```python
from build123d import *

# Parameters (mm, degrees)
SKETCH1_W                    = 38.1
SKETCH1_H                    = 53.34
BOSS_EXTRUDE1_DEPTH          = 1.5875
EDGE_FLANGE1_STRIP_W         = 9.525
EDGE_FLANGE1_STRIP_H         = 1.5875
EDGE_FLANGE1_STRIP_CUT_DEPTH = 38.1
EDGE_FLANGE1_DEPTH           = 38.1
CUT_EXTRUDE1_REACH           = 40.731
SKETCH9_R                    = 2.54
CUT_EXTRUDE2_REACH           = 61.758
SKETCH11_R                   = 2.54


# Sheet-metal steps are written as plain solids
with BuildPart() as part:
    # Sketch1 → Boss-Extrude1 (new body)
    with BuildSketch(Plane(origin=(0, 0, 0), x_dir=(1, 0, 0), z_dir=(0, 1, 0))):
        Rectangle(SKETCH1_W, SKETCH1_H)
    extrude(amount=BOSS_EXTRUDE1_DEPTH)

    # Edge-Flange1 strip (across the edge) → Edge-Flange1 strip cut (cut)
    with BuildSketch(Plane(origin=(19.05, 0, 26.67), x_dir=(0, 0, -1), z_dir=(-1, 0, 0))):
        with Locations((-1.5875, -0.79375)):
            Rectangle(EDGE_FLANGE1_STRIP_W, EDGE_FLANGE1_STRIP_H)
    extrude(amount=EDGE_FLANGE1_STRIP_CUT_DEPTH, mode=Mode.SUBTRACT)

    # Edge-Flange1 section (across the edge) → Edge-Flange1 (add)
    with BuildSketch(Plane(origin=(19.05, 0, 26.67), x_dir=(0, 0, -1), z_dir=(-1, 0, 0))):
        with BuildLine():
            Line((0, 1.5875), (0, 19.05))
            Line((0, 19.05), (1.5875, 19.05))
            Line((1.5875, 19.05), (1.5875, 1.5875))
            ThreePointArc((1.5875, 1.5875), (2.052467985, 0.464967985), (3.175, 0))
            Line((3.175, 0), (3.175, -1.5875))
            ThreePointArc((3.175, -1.5875), (0.92993597, -0.65756403), (0, 1.5875))
        make_face()
    extrude(amount=EDGE_FLANGE1_DEPTH)

    # Sketch9 → Cut-Extrude1 (cut, up to next)
    with BuildSketch(Plane(origin=(0, 1.5875, 0), x_dir=(1, 0, 0), z_dir=(0, 1, 0)), mode=Mode.PRIVATE) as cut_extrude1_sk1:
        with Locations(Location((9.813099354, 13.0175, 0), (0, 0, 270))):
            Circle(SKETCH9_R)
    cut_extrude1_tool1 = extrude(cut_extrude1_sk1.sketch, amount=-CUT_EXTRUDE1_REACH, mode=Mode.PRIVATE) & part.part
    # Sketch9 → Cut-Extrude1 (cut, up to next)
    with BuildSketch(Plane(origin=(0, 1.5875, 0), x_dir=(1, 0, 0), z_dir=(0, 1, 0)), mode=Mode.PRIVATE) as cut_extrude1_sk2:
        with Locations(Location((-9.236900646, 13.0175, 0), (0, 0, 270))):
            Circle(SKETCH9_R)
    cut_extrude1_tool2 = extrude(cut_extrude1_sk2.sketch, amount=-CUT_EXTRUDE1_REACH, mode=Mode.PRIVATE) & part.part
    add(cut_extrude1_tool1.solids().sort_by_distance((9.813099, 1.5875, -13.0175))[0], mode=Mode.SUBTRACT)
    add(cut_extrude1_tool2.solids().sort_by_distance((-9.236901, 1.5875, -13.0175))[0], mode=Mode.SUBTRACT)

    # Sketch11 → Cut-Extrude2 (cut, up to next)
    with BuildSketch(Plane.XY.offset(26.67), mode=Mode.PRIVATE) as cut_extrude2_sk1:
        with Locations((-9.398, -9.398)):
            Circle(SKETCH11_R)
    cut_extrude2_tool1 = extrude(cut_extrude2_sk1.sketch, amount=-CUT_EXTRUDE2_REACH, mode=Mode.PRIVATE) & part.part
    # Sketch11 → Cut-Extrude2 (cut, up to next)
    with BuildSketch(Plane.XY.offset(26.67), mode=Mode.PRIVATE) as cut_extrude2_sk2:
        with Locations((9.398, -9.398)):
            Circle(SKETCH11_R)
    cut_extrude2_tool2 = extrude(cut_extrude2_sk2.sketch, amount=-CUT_EXTRUDE2_REACH, mode=Mode.PRIVATE) & part.part
    add(cut_extrude2_tool1.solids().sort_by_distance((-9.398, -9.398, 26.67))[0], mode=Mode.SUBTRACT)
    add(cut_extrude2_tool2.solids().sort_by_distance((9.398, -9.398, 26.67))[0], mode=Mode.SUBTRACT)


solid = part.part
```
Input: part model. Units: mm. Frame: model coordinates. A direction names the side the tool comes from. Coordinates: 2 decimals unless noted, no trailing zeros. Loops run counter-clockwise (first coordinate to the right, second up) from the corner with the lowest first, then second, coordinate; pieces in that order, holes last. Notation, with made-up numbers: M 14.25,89 L 45.25,89 A18 cw 45.25,111 Z; hole C 62,16.25 d11. An arc over 180 degrees is marked long. Use a Markdown table: item, result. Add a question column.
1) Draft query along X for faces 3 (the cylindrical face through (-10.782, 0.805, -15.033)), 4 (the flat face through (0, -19.05, 26)), 5 (the flat face through (-19.05, 0.4, 7.8)), 6 (the cylindrical face through (11.821, -8.635, 25.887)). Return one class per face: +X half, -X half, draft (parallel to the pull), parting line (faces both ways), or undercut.
2) Set-up query: faces 1 (the flat face through (0, -10, 25.083)), 2 (the flat face through (0, 1, -26.67)). Return all of +Z, -Z, +X, -X, +Y, -Y with unobstructed straight access to the full face (end or side cutting, diameter ignored); none if empty.
3) Pin query (flat end, axial travel): P1, Ø1, axis at x = 15, z = 17.5, coming from the -Y side; P2, Ø5, axis at x = -6.5, y = -13, coming from the -Z side. Return the tip coordinate at first contact, or that it passes through.
4) Section B-B, the plane y = -10.75. Return the cut outline in (x, z).
5) Section D-D, the plane z = 0. Return the cut outline in (x, y).
6) Line query: L1, parallel to Y at x = -8, z = -21; L2, parallel to Z at x = 2, y = -11.5; L3, parallel to Z at x = -7.5, y = -1. Output: solid intervals per line, ascending. Write a range as from..to.
7) Section A-A, the plane x = 9. Give the number of separate pieces and of enclosed holes in the cut face, plus the area to 3 significant figures.
Answer below:
| question | item | result |
|---|---|---|
| 1 | face 3 | undercut |
| 1 | face 4 | draft |
| 1 | face 5 | -X half |
| 1 | face 6 | undercut |
| 2 | face 1 | -Z, +X, -X, -Y |
| 2 | face 2 | -Z, +X, -X, +Y, -Y |
| 3 | P1 | y = 0 |
| 3 | P2 | z = 25.08 |
| 4 | outline | M -19.05,25.08 L -11.55,25.08 L -11.55,26.67 L -19.05,26.67 Z; M -7.25,25.08 L 7.25,25.08 L 7.25,26.67 L -7.25,26.67 Z; M 11.55,25.08 L 19.05,25.08 L 19.05,26.67 L 11.55,26.67 Z |
| 5 | outline | M -19.05,0 L 19.05,0 L 19.05,1.59 L -19.05,1.59 Z |
| 6 | L1 | 0..1.59 |
| 6 | L2 | 25.08..26.67 |
| 6 | L3 | 24.97..26.62 |
| 7 | separate pieces | 3 |
| 7 | enclosed holes | 0 |
| 7 | area | 97.7 mm2 |
